```python
from build123d import *

# Parameters (mm, degrees)
SKETCH1_R           = 14.278677311
SKETCH1_R_2         = 2.261632511
BOSS_EXTRUDE1_DEPTH = 19
SKETCH1_3_R         = 14.278677311
SKETCH1_3_R_2       = 2.261632511
CUT_EXTRUDE1_DEPTH  = 18
DOME1_FACE_RADIUS   = 14.278677311
DOME1_HEIGHT        = 4
DOME2_FACE_RADIUS   = 14.278677311
DOME2_HEIGHT        = 4


with BuildPart() as part:
    # Sketch1 → Boss-Extrude1 (new, symmetric)
    with BuildSketch(Plane(origin=(0, 0, 0), x_dir=(1, 0, 0), z_dir=(0, 1, 0))):
        with Locations(Location((0, 0, 0), (0, 0, 270))):
            Circle(SKETCH1_R)
        Circle(SKETCH1_R_2, mode=Mode.SUBTRACT)
        Circle(SKETCH1_R_2)
    extrude(amount=BOSS_EXTRUDE1_DEPTH, both=True)

    # Sketch1<3> → Cut-Extrude1 (cut, symmetric)
    with BuildSketch(Plane(origin=(0, 0, 0), x_dir=(1, 0, 0), z_dir=(0, 1, 0))):
        with Locations(Location((0, 0, 0), (0, 0, 270))):
            Circle(SKETCH1_3_R)
        with Locations(Location((0, 0, 0), (0, 0, 270))):
            Circle(SKETCH1_3_R_2, mode=Mode.SUBTRACT)
    extrude(amount=CUT_EXTRUDE1_DEPTH, both=True, mode=Mode.SUBTRACT)

    # Dome1: a dome of height H over a round flat face of radius A is a cap of a sphere of radius (A * A + H * H) / (2 * H)
    dome1_r = (DOME1_FACE_RADIUS * DOME1_FACE_RADIUS + DOME1_HEIGHT * DOME1_HEIGHT) / (2 * DOME1_HEIGHT)
    dome1_base = Plane((0, -19, 0), z_dir=(0, -1, 0))
    with Locations(dome1_base.offset(DOME1_HEIGHT - dome1_r)):
        dome1_ball = Sphere(dome1_r, mode=Mode.PRIVATE)
    add(split(dome1_ball, bisect_by=dome1_base, keep=Keep.TOP, mode=Mode.PRIVATE))

    # Dome2: a dome of height H over a round flat face of radius A is a cap of a sphere of radius (A * A + H * H) / (2 * H)
    dome2_r = (DOME2_FACE_RADIUS * DOME2_FACE_RADIUS + DOME2_HEIGHT * DOME2_HEIGHT) / (2 * DOME2_HEIGHT)
    dome2_base = Plane((0, 19, 0), z_dir=(0, 1, 0))
    with Locations(dome2_base.offset(DOME2_HEIGHT - dome2_r)):
        dome2_ball = Sphere(dome2_r, mode=Mode.PRIVATE)
    add(split(dome2_ball, bisect_by=dome2_base, keep=Keep.TOP, mode=Mode.PRIVATE))


solid = part.part
```
Can you work these out from the model? Positions are in its coordinate system, mm. A direction names the side the tool comes from. Round coordinates to 2 decimals unless told otherwise and drop trailing zeros. Loops run counter-clockwise (first coordinate to the right, second up) from the corner with the lowest first, then second, coordinate; pieces in that order, holes last. Notation, with made-up numbers: M 20,-8 L 67,-8 A17 ccw 67,13 Z; hole C -29.75,75.5 d6. An arc over 180 degrees is marked long. Answer as a JSON object with one key per item and string values. Group by question number.
Q1. Will these pins go through, and if not, where does the flat tip stop? pin 1 (12 mm diameter, centred on x = 4, z = -10.5, fed in from -Y); pin 2 (2 mm diameter, centred on x = 3.5, z = -9, fed in from -Y); pin 3 (8.5 mm diameter, centred on x = 4.5, z = 3.5, fed in from +Y).
Q2. On a 3-axis mill with a long thin cutter (end or side, diameter ignored), from which of +Z, -Z, +X, -X, +Y, -Y can I reach the whole of each face in a straight line? I mean faces 1 (the cylindrical face through (-1.38, -0.25, -1.79)), 2 (the cylindrical face through (-5.47, -18.49, 13.19)). Say none if no direction works.
Q3. Imagine slicing it at C-C, the plane x = 5.25. Please give me the cut outline in (y, z).
Q4. Please list where these lines run through material, in increasing order: L1, parallel to Y at x = -7.5, z = 10; L2, parallel to Y at x = 8.25, z = -5.5; L3, parallel to X at y = -10.5, z = -1.75.
Q5. We'd pull the mould along Y, two halves only. Please class faces 3 (the cylindrical face through (-5.47, 18.51, 13.19)), 4 (the flat face through (0, 18, 3)): +Y half, -Y half, draft (parallel to the pull), parting line (faces both ways), or undercut.
Q6. Imagine slicing it at D-D, the plane z = -9.75. Please give me the cut outline in (x, y), then the cut area to 3 significant figures.
Q7. Imagine slicing it at A-A, the plane x = 0. Please give me the cut outline in (y, z), then the cut area to 3 significant figures.
Q8. Imagine slicing it at B-B, the plane z = 0. Please give me the cut outline in (x, y), then the cut area to 3 significant figures.
Findings:
{
 "1": {"pin 1": "stops at y = -22.5", "pin 2": "stops at y = -21.6", "pin 3": "stops at y = 22.96"},
 "2": {"face 1": "none", "face 2": "+Y, -Y"},
 "3": {"outline": "M -19,-13.28 L -18,-13.28 L -18,13.28 L -19,13.28 A26.98 ccw Z; M 18,-13.28 L 19,-13.28 A26.98 ccw 19,13.28 L 18,13.28 Z"},
 "4": {"L1": "y = -19.99 to -18, 18 to 19.99", "L2": "y = -21.15 to -18, 18 to 21.15", "L3": "x = -1.43 to 1.43"},
 "5": {"face 3": "draft", "face 4": "undercut"},
 "6": {"outline": "M -10.43,-19 A25.7 ccw 10.43,-19 L 10.43,-18 L -10.43,-18 Z; M -10.43,18 L 10.43,18 L 10.43,19 A25.7 ccw -10.43,19 Z", "area": "104 mm2"},
 "7": {"outline": "M -19,-14.28 L -18,-14.28 L -18,-2.26 L 18,-2.26 L 18,-14.28 L 19,-14.28 A27.49 ccw 19,14.28 L 18,14.28 L 18,2.26 L -18,2.26 L -18,14.28 L -19,14.28 A27.49 ccw Z", "area": "375 mm2"},
 "8": {"outline": "M -14.28,-19 A27.49 ccw 14.28,-19 L 14.28,-18 L 2.26,-18 L 2.26,18 L 14.28,18 L 14.28,19 A27.49 ccw -14.28,19 L -14.28,18 L -2.26,18 L -2.26,-18 L -14.28,-18 Z", "area": "375 mm2"}
}
